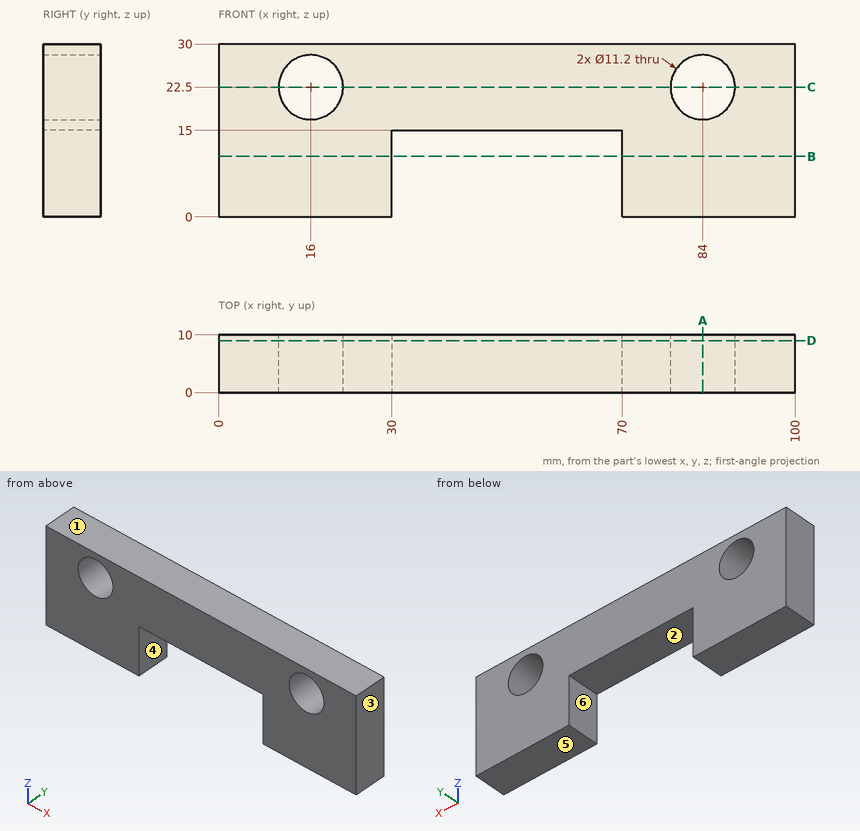
Study the drawing (mm; zero at the part's minimum x, y, z) and answer. A direction names the side the tool comes from. Round coordinates to 2 decimals unless told otherwise and drop trailing zeros. Loops run counter-clockwise (first coordinate to the right, second up) from the corner with the lowest first, then second, coordinate; pieces in that order, holes last. Notation, with made-up numbers: (41.5, 44.25) - (57.5, 44.25) arc R12 cw to (57.5, 57.25) - close; hole circle Ø2 at (70.5, 33.25). An arc over 180 degrees is marked (long way). Use one line per item in the form item = value. Start each with the question number.
1. Consider line 1 (X direction, y = 5, z = 11.75); line 2 (Z direction, x = 16, y = 6.5); line 3 (X direction, y = 4.5, z = 25.5). Determine where each line is inside the solid, lowest interval first. Write a range as [from, to].
2. The part is cut by section D-D on y = 9. Determine the outline of the cut face in (x, z), then the cut area to 3 significant figures.
3. The part is cut by section A-A on x = 84. Determine the outline of the cut face in (y, z), then the cut area to 3 significant figures.
4. A tool of negligible diameter and unlimited length cuts with its end or side. For the marked faces 1 and 2, from which of +Z, -Z, +X, -X, +Y, -Y can it reach the whole face along a straight path? Write none if from no direction.
5. Given pin 1 Ø10 at (x, z) = (16, 22.5) entering from +Y; pin 2 Ø3 at (x, y) = (52.5, 4) entering from -Z, each flat-ended and moving along its own axis, determine where each tip first touches the part or whether it passes through.
6. The part is cut by section C-C on z = 22.5. Determine the outline of the cut face in (x, y), then the cut area to 3 significant figures.
7. The part is cut by section B-B on z = 10.5. Determine the outline of the cut face in (x, y).
8. For a pull along X with two mould halves and no side action, classify the marked faces 3, 4, 5 and 6 as pulls with the +X half, pulls with the -X half, needs draft (parallel to the pull), parting line crosses it, or undercut.
Geometry check:
q1.line_1 = [0, 30], [70, 100]
q1.line_2 = [0, 16.9], [28.1, 30]
q1.line_3 = [0, 11.27], [20.73, 79.27], [88.73, 100]
q2.outline = (0, 0) - (30, 0) - (30, 15) - (70, 15) - (70, 0) - (100, 0) - (100, 30) - (0, 30) - close; hole circle Ø11.2 at (16, 22.5); hole circle Ø11.2 at (84, 22.5)
q2.area = 2,200 mm^2
q3.outline = (0, 0) - (10, 0) - (10, 16.9) - (0, 16.9) - close; (0, 28.1) - (10, 28.1) - (10, 30) - (0, 30) - close
q3.area = 188 mm^2
q4.face_1 = +Z, +X, -X, +Y, -Y
q4.face_2 = -Z, +Y, -Y
q5.pin_1 = through
q5.pin_2 = 15
q6.outline = (0, 0) - (10.4, 0) - (10.4, 10) - (0, 10) - close; (21.6, 0) - (78.4, 0) - (78.4, 10) - (21.6, 10) - close; (89.6, 0) - (100, 0) - (100, 10) - (89.6, 10) - close
q6.area = 776 mm^2
q7.outline = (0, 0) - (30, 0) - (30, 10) - (0, 10) - close; (70, 0) - (100, 0) - (100, 10) - (70, 10) - close
q8.face_3 = pulls with the +X half
q8.face_4 = undercut
q8.face_5 = needs draft
q8.face_6 = undercut
